from build123d import *

# Parameters (mm, degrees)
F1_DEPTH = 19.05
F2_DEPTH = 6.35


# Not quite as in the source:
# - a length typed as a fraction of an inch, garbled in the dataset ("3 / 203.2 mm" for 3/8 in), is restored


with BuildPart() as f1:
    # F0 (on Top) → F1 (new body)
    with BuildSketch(Plane.XY):
        with BuildLine():
            Line((927.1, 0), (12.7, 0))
            ThreePointArc((12.7, 0), (12.1376302063, -2.6126302063), (10.5501302063, -4.7625))
            Line((10.5501302063, -4.7625), (927.1, -4.7625))
            Line((927.1, -4.7625), (927.1, 0))
        make_face()
        with BuildLine():
            Line((927.1, -4.7625), (10.5501302063, -4.7625))
            ThreePointArc((10.5501302063, -4.7625), (2.8938151032, -12.4188151032), (-4.7625, -4.7625))
            Line((-4.7625, -4.7625), (-4.7625, 139.7))
            Line((-4.7625, 139.7), (-76.2, 139.7))
            Line((-76.2, 139.7), (-76.2, -76.2))
            Line((-76.2, -76.2), (927.1, -76.2))
            Line((927.1, -76.2), (927.1, -4.7625))
        make_face()
        with BuildLine():
            ThreePointArc((-4.7625, -4.7625), (2.8938151032, -12.4188151032), (10.5501302063, -4.7625))
            ThreePointArc((10.5501302063, -4.7625), (3.7373697937, -5.7876302063), (0, 0))
            Line((0, 0), (0, 139.7))
            Line((0, 139.7), (-4.7625, 139.7))
            Line((-4.7625, 139.7), (-4.7625, -4.7625))
        make_face()
    extrude(amount=-F1_DEPTH)

    # F0 (on Top) → F2 (join)
    with BuildSketch(Plane.XY):
        with BuildLine():
            Line((927.1, -4.7625), (10.5501302063, -4.7625))
            ThreePointArc((10.5501302063, -4.7625), (2.8938151032, -12.4188151032), (-4.7625, -4.7625))
            Line((-4.7625, -4.7625), (-4.7625, 139.7))
            Line((-4.7625, 139.7), (-76.2, 139.7))
            Line((-76.2, 139.7), (-76.2, -76.2))
            Line((-76.2, -76.2), (927.1, -76.2))
            Line((927.1, -76.2), (927.1, -4.7625))
        make_face()
    extrude(amount=F2_DEPTH)


solid = f1.part
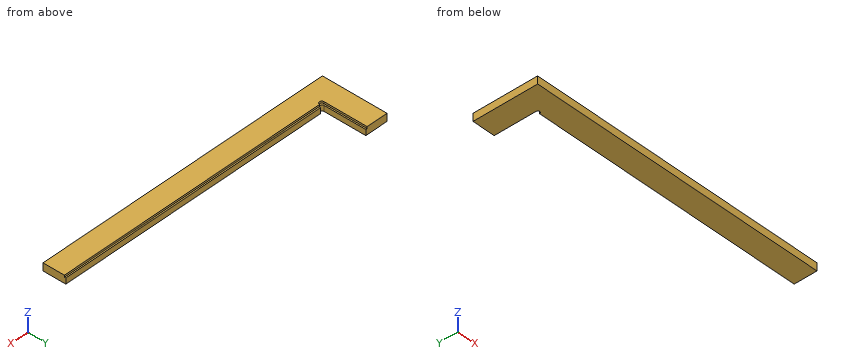
Check sheet for the modelled part. Datum: model origin and axes. Units: mm. Round coordinates to 2 decimals unless told otherwise and drop trailing zeros. Order: outer loops, then holes, each group sorted by start corner. A loop starts at its lowest first (then second) coordinate and runs counter-clockwise, first axis right, second up. Notation, with made-up numbers: M 78.25,-37 L 116.25,-37 A29 ccw 116.25,-9 Z; hole C 22,65 d8. An arc over 180 degrees is marked long. One line per item, written item: value. Start each with the question number.
1. Section check A-A on z = -13.25. Enter the section's corners in (x, y).
2. Section check B-B on y = 34.5. Enter the section's corners in (x, z), and give its area (3 significant figures).
3. Gauge pin test, flat ends, axial feed: P1, Ø7, axis at x = 263, z = 4.5, coming from the +Y side; P2, Ø5, axis at y = 74, z = 4, coming from the +X side; P3, Ø12, axis at y = 72, z = -14, coming from the +X side. Record the tip position at first contact, or that the pin passes through.
4. Scan lines: line 1 along Y through (x, z) = (601, -9.5); line 2 along X through (y, z) = (-10.5, 1.5). Record each from-to range of solid material in increasing order.
Results found:
1. outline: M -76.2,-76.2 L 927.1,-76.2 L 927.1,0 L 12.7,0 A6.35 cw 0,0 L 0,139.7 L -76.2,139.7 Z
2. outline: M -76.2,-19.05 L 0,-19.05 L 0,0 L -4.76,0 L -4.76,6.35 L -76.2,6.35 Z
2. area: 1,910 mm^2
3. P1: y = -4.76
3. P2: x = -4.76
3. P3: x = 0
4. line 1: -76.2 to 0
4. line 2: -76.2 to -2.18, 7.96 to 927.1
